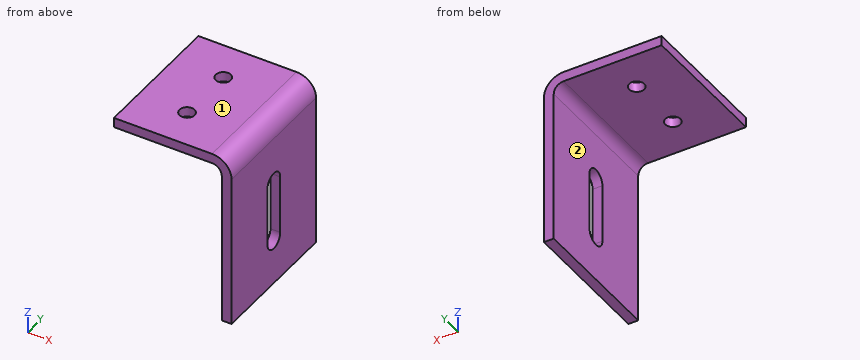
from build123d import *

# Parameters (mm, degrees)
SKETCH1_W                    = 38.1
SKETCH1_H                    = 44.45
BASE_FLANGE1_DEPTH           = 3.175
EDGE_FLANGE1_STRIP_W         = 19.05
EDGE_FLANGE1_STRIP_H         = 3.175
EDGE_FLANGE1_STRIP_CUT_DEPTH = 44.45
EDGE_FLANGE1_DEPTH           = 44.45
SKETCH9_R                    = 2.4511
CUT_EXTRUDE1_DEPTH           = 61.377066247
CUT_EXTRUDE3_DEPTH           = 70.625037081


# Sheet-metal steps are written as plain solids
with BuildPart() as part:
    # Sketch1 → Base-Flange1 (new body)
    with BuildSketch(Plane.XY):
        Rectangle(SKETCH1_W, SKETCH1_H)
    extrude(amount=-BASE_FLANGE1_DEPTH)

    # Edge-Flange1 strip (across the edge) → Edge-Flange1 strip cut (cut)
    with BuildSketch(Plane(origin=(19.05, 22.225, -3.175), x_dir=(-1, 0, 0), z_dir=(0, -1, 0))):
        with Locations((-3.175, -1.5875)):
            Rectangle(EDGE_FLANGE1_STRIP_W, EDGE_FLANGE1_STRIP_H)
    extrude(amount=EDGE_FLANGE1_STRIP_CUT_DEPTH, mode=Mode.SUBTRACT)

    # Edge-Flange1 section (across the edge) → Edge-Flange1 (add)
    with BuildSketch(Plane(origin=(19.05, 22.225, -3.175), x_dir=(-1, 0, 0), z_dir=(0, -1, 0))):
        with BuildLine():
            Line((0, 3.175), (0, 52.8066))
            Line((0, 52.8066), (3.175, 52.8066))
            Line((3.175, 52.8066), (3.175, 3.175))
            ThreePointArc((3.175, 3.175), (4.10493597, 0.92993597), (6.35, 0))
            Line((6.35, 0), (6.35, -3.175))
            ThreePointArc((6.35, -3.175), (1.859871939, -1.315128061), (0, 3.175))
        make_face()
    extrude(amount=EDGE_FLANGE1_DEPTH)

    # Sketch9 → Cut-Extrude1 (cut, through all)
    with BuildSketch(Plane(origin=(0, 0, -3.175), x_dir=(-1, 0, 0), z_dir=(0, 0, -1))):
        with Locations((3.175, 9.525)):
            Circle(SKETCH9_R)
        with Locations((3.175, -9.525)):
            Circle(SKETCH9_R)
    extrude(amount=-CUT_EXTRUDE1_DEPTH, mode=Mode.SUBTRACT)

    # Sketch12 → Cut-Extrude3 (cut, through all)
    with BuildSketch(Plane.ZY.offset(-15.875)):
        with BuildLine():
            Line((-40.6908, 3.3734375), (-21.6408, 3.3734375))
            ThreePointArc((-21.6408, 3.3734375), (-18.2673625, 0), (-21.6408, -3.3734375))
            Line((-21.6408, -3.3734375), (-40.6908, -3.3734375))
            ThreePointArc((-40.6908, -3.3734375), (-44.0642375, 0), (-40.6908, 3.3734375))
        make_face()
    extrude(amount=-CUT_EXTRUDE3_DEPTH, mode=Mode.SUBTRACT)


solid = part.part
Design review of the part built by this model. Coordinates are the model's own, in mm. Face numbers are marked on the shaded views. A direction names the side the tool comes from. Round coordinates to 2 decimals unless told otherwise and drop trailing zeros. Loops run counter-clockwise (first coordinate to the right, second up) from the corner with the lowest first, then second, coordinate; pieces in that order, holes last. Notation, with made-up numbers: (-4.75, 7.5) - (12.25, 7.5) arc R21 cw to (12.25, 25.5) - close; hole circle Ø4 at (31, 28). An arc over 180 degrees is marked (long way). One line per item, written item: value. Start each with the question number.
1) For the marked faces 1 and 2, list the 3-axis set-ups (+Z, -Z, +X, -X, +Y, -Y) from which the entire face can be reached by the end or side of a thin tool; tool diameter is ignored.
2) Consider section D-D on y = 4.5. Give the boundary of the cut face in (x, z) (3 decimals).
3) Consider section B-B on y = 0. Give the boundary of the cut face in (x, z) (3 decimals), then the cut area to 3 significant figures.
4) Consider section A-A on z = -23.5. Give the boundary of the cut face in (x, y) (3 decimals), then the cut area to 3 significant figures.
5) Consider section C-C on x = 17.5. Give the boundary of the cut face in (y, z) (3 decimals).
6) Insertion check: pin 1 Ø1 at (y, z) = (0.5, -17) entering from -X (3 decimals); pin 2 Ø2 at (x, y) = (-3.5, 17) entering from -Z (3 decimals). Each pin has a flat end and moves straight along its axis. Give the tip position at first contact, or say it passes through.
7) To check wall thickness, follow L1, parallel to X at y = 5, z = -6.5 (3 decimals); L2, parallel to Z at x = -8.5, y = 2 (3 decimals); L3, parallel to X at y = 1, z = -3. State the ranges of each line that lie inside material, in increasing order. Write a range as from..to.
Reported:
1. face 1: +Z, +X, -X, +Y, -Y
1. face 2: -Z, -X, +Y, -Y
2. outline: (-19.05, -3.175) - (12.7, -3.175) arc R3.175 cw to (15.875, -6.35) - (15.875, -55.982) - (19.05, -55.982) - (19.05, -6.35) arc R6.35 ccw to (12.7, 0) - (-19.05, 0) - close
3. outline: (-19.05, -3.175) - (12.7, -3.175) arc R3.175 cw to (15.875, -6.35) - (15.875, -18.267) - (19.05, -18.267) - (19.05, -6.35) arc R6.35 ccw to (12.7, 0) - (-19.05, 0) - close; (15.875, -55.982) - (19.05, -55.982) - (19.05, -44.064) - (15.875, -44.064) - close
3. area: 200 mm^2
4. outline: (15.875, -22.225) - (19.05, -22.225) - (19.05, -3.373) - (15.875, -3.373) - close; (15.875, 3.373) - (19.05, 3.373) - (19.05, 22.225) - (15.875, 22.225) - close
4. area: 120 mm^2
5. outline: (-22.225, -55.982) - (22.225, -55.982) - (22.225, -2.193) - (-22.225, -2.193) - close; hole (-3.373, -40.691) arc R3.373 ccw to (3.373, -40.691) - (3.373, -21.641) arc R3.373 ccw to (-3.373, -21.641) - close
6. pin 1: stops at x = 15.875
6. pin 2: stops at z = -3.175
7. L1: x = 15.875..19.05
7. L2: z = -3.175..0
7. L3: x = -19.05..18.09
